Autodesk Inventor part; units mm, degrees
ref_plane "YZ Plane" through (0, 0, 0) normal (1, 0, 0) x (0, 1, 0)
ref_plane "XZ Plane" through (0, 0, 0) normal (0, 1, 0) x (-1, 0, 0)
ref_plane "XY Plane" through (0, 0, 0) normal (0, 0, 1) x (1, 0, 0)
sketch "Sketch1" plane through (0, 0, 0) normal (0, 0, 1) x (1, 0, 0)
  line L0 (0, 0) -> (36, 0)
  line L1 (36, 0) -> (36, 62)
  line L2 (36, 62) -> (0, 62)
  line L3 (0, 62) -> (0, 0)
  line L4 (-2.5, -2.5) -> (38.5, -2.5)
  line L5 (38.5, -2.5) -> (38.5, 64.5)
  line L6 (38.5, 64.5) -> (-2.5, 64.5)
  line L7 (-2.5, 64.5) -> (-2.5, -2.5)
  dimension "d0" = 36
  dimension "d1" = 62
  dimension "d2" = 2.5
extrude "Extrusion1" add sketch "Sketch1" along normal blind 17 contours L3 L2 L1 L0 | L7 L6 L5 L4
sketch "Sketch2" plane through (0, 0, 17) normal (0, 0, 1) x (1, 0, 0)
  line L0 (-2.5, -2.5) -> (38.5, -2.5)
  line L1 (38.5, -2.5) -> (38.5, 64.5)
  line L2 (38.5, 64.5) -> (-2.5, 64.5)
  line L3 (-2.5, 64.5) -> (-2.5, -2.5)
  line L4 (0, 0) -> (36, 0)
  line L5 (36, 0) -> (36, 62)
  line L6 (36, 62) -> (0, 62)
  line L7 (0, 62) -> (0, 0)
  point P0 (0, 0)
  dimension "d5" = 2.5
extrude "Extrusion2" cut sketch "Sketch2" against normal blind 14 contours L7 L6 L5 L4
sketch "Sketch3" plane through (0, 0, 17) normal (0, 0, 1) x (1, 0, 0)
  line L0 (36, 0) -> (0, 0)
  line L1 (36, 62) -> (36, 0)
  line L2 (0, 62) -> (36, 62)
  line L3 (0, 0) -> (0, 62)
  line L4 (10, 61.5) -> (26, 61.5)
  line L5 (35.5, 52) -> (35.5, 10)
  line L6 (26, 0.5) -> (10, 0.5)
  line L7 (0.5, 10) -> (0.5, 52)
  line L8 (0, 52) -> (0.5, 52)
  line L9 (35.5, 52) -> (36, 52)
  line L10 (10, 61.5) -> (10, 62)
  line L11 (26, 62) -> (26, 61.5)
  line L12 (36, 10) -> (35.5, 10)
  line L13 (26, 0.5) -> (26, 0)
  line L14 (10, 0) -> (10, 0.5)
  line L15 (0.5, 10) -> (0, 10)
  point P0 (0, 0)
  dimension "d9" = 0.5
extrude "Extrusion3" add sketch "Sketch3" against normal blind 1 contours L0 L14 L6 L13 | L12 L5 L9 L1 | L3 L8 L7 L15 | L11 L4 L10 L2
fillet "Fillet1" radius 2 4 edges at (0.5, 31, 16) (18, 61.5, 16) (35.5, 31, 16) (18, 0.5, 16)
sketch "Sketch4" plane through (-2.5, 64.5, 0) normal (0, 1, 0) x (1, 0, 0)
  line L0 (41, -17) -> (0, -17)
  line L1 (20.5, -17) -> (27.5, -17)
  circle A0 centre (27.5, -17) radius 2.5
  point P0 (2.5, 0)
  dimension "d13" = 7
  dimension "d14" = 5
extrude "Extrusion4" cut sketch "Sketch4" against normal blind 4
properties part number "feeder_encolsure"
The model under review builds one solid part; all positions refer to its coordinate system, in mm. A direction names the side the tool comes from. Coordinates: 2 decimals unless noted, no trailing zeros. Write each loop counter-clockwise with the first axis right and the second up, starting at its lowest first coordinate (ties: lowest second). Pieces come first, ordered by that corner, then holes. Notation, with made-up numbers: M 67.25,77.25 L 91.25,77.25 A12 cw 91.25,94.25 Z; hole C 35.5,-19.5 d10. An arc over 180 degrees is marked long. Put each result on its own line as item: value.
1) Draft analysis for pull direction Z (two halves, no side actions). For faces 3 (the flat face through (18, 64.5, 8)), 4 (the flat face through (18, 62, 10)), 5 (the flat face through (18, 31, 0)), 6 (the cylindrical face through (25.1, 63, 14.5)), state which applies: released by +Z, released by -Z, zero draft, split by the parting line, or undercut.
Computed:
face 3: zero draft
face 4: undercut
face 5: released by -Z
face 6: released by +Z
2) For faces 1 (the flat face through (0, 31, 10)), 2 (the flat face through (38.5, 31, 8)), list the 3-axis set-ups (+Z, -Z, +X, -X, +Y, -Y) from which the entire face can be reached by the end or side of a thin tool; tool diameter is ignored.
Computed:
face 1: none
face 2: +Z, -Z, +X, +Y, -Y
3) Clearance check with flat-ended pins moving along their axes: pin 1 Ø11 at (x, y) = (11.5, 22) entering from +Z; pin 2 Ø4 at (x, y) = (21.5, 35) entering from -Z. State where each tip first meets the part, or that it passes through.
Computed:
pin 1: stops at z = 3
pin 2: stops at z = 0
4) Add section D-D on x = 11. Give the boundary of the cut face in (y, z).
Computed:
outline: M -2.5,0 L 64.5,0 L 64.5,17 L 61.5,17 A2 ccw 62,16 L 62,3 L 0,3 L 0,16 A2 ccw 0.5,17 L -2.5,17 Z
5) Add section B-B on z = 10.25. Give the boundary of the cut face in (x, y).
Computed:
outline: M -2.5,-2.5 L 38.5,-2.5 L 38.5,64.5 L -2.5,64.5 Z; hole M 0,0 L 36,0 L 36,62 L 0,62 Z
6) Add section A-A on y = 41.5. Give the boundary of the cut face in (x, z), then the cut area to 3 significant figures.
Computed:
outline: M -2.5,0 L 38.5,0 L 38.5,17 L 35.5,17 A2 ccw 36,16 L 36,3 L 0,3 L 0,16 A2 ccw 0.5,17 L -2.5,17 Z
area: 194 mm2
7) Add section C-C on x = 5. Give the boundary of the cut face in (y, z), then the cut area to 3 significant figures.
Computed:
outline: M -2.5,0 L 64.5,0 L 64.5,17 L 62,17 L 62,3 L 0,3 L 0,17 L -2.5,17 Z
area: 271 mm2
8) Wall thickness on probe 1 along Y at (x, z) = (12.5, 9); probe 2 along X at (y, z) = (47, 10); probe 3 along Z at (x, y) = (23.5, 38): over which ranges is each line inside the solid? List them lowest first. Write a range as [from, to].
Computed:
probe 1: y = [-2.5, 0], [62, 64.5]
probe 2: x = [-2.5, 0], [36, 38.5]
probe 3: z = [0, 3]
